Build history of the part. All positions in model axes, mm. A direction names the side the tool comes from. Give positions to 0.01 mm unless a question says otherwise; leave off trailing zeros. Write each loop counter-clockwise with the first axis right and the second up, starting at its lowest first coordinate (ties: lowest second). Pieces come first, ordered by that corner, then holes.
Autodesk Inventor part; units mm, degrees
ref_plane "YZ Plane" through (0, 0, 0) normal (1, 0, 0) x (0, 1, 0)
ref_plane "XZ Plane" through (0, 0, 0) normal (0, 1, 0) x (-1, 0, 0)
ref_plane "XY Plane" through (0, 0, 0) normal (0, 0, 1) x (1, 0, 0)
sketch "Sketch1" plane through (0, 0, 0) normal (0, 1, 0) x (-1, 0, 0)
  line L0 (-24.2, -24.2) -> (24.2, -24.2)
  line L1 (24.2, -24.2) -> (24.2, 24.2)
  line L2 (24.2, 24.2) -> (-24.2, 24.2)
  line L3 (-24.2, 24.2) -> (-24.2, -24.2)
  point P0 (0, 0)
  point P1 (0, 24.2)
  point P2 (-24.2, 0)
  dimension "d0" = 48.4
  dimension "d2" = 48.4
extrude "Extrusion1" add sketch "Sketch1" along normal blind 45
sketch "Sketch2" plane through (0, 45, 0) normal (0, 1, 0) x (1, 0, 0)
  circle A0 centre (0, 0) radius 21
  dimension "d5" = 42
extrude "Extrusion2" add sketch "Sketch2" along normal blind 12.5
sketch "Sketch3" plane through (0, 57.5, 0) normal (0, 1, 0) x (1, 0, 0)
  circle A0 centre (0, 0) radius 21
  circle A1 centre (0, 0) radius 20.1325
extrude "Extrusion3" add sketch "Sketch3" along normal blind 9 contours A1
chamfer "Chamfer1" distance 2 distance2 9 1 edges at (-20.1325, 66.5, 0) measured on face at (-5.7471, 66.5, 1.5127)
sketch "Sketch4" plane through (0, 66.5, 0) normal (0, 1, 0) x (1, 0, 0)
  circle A0 centre (0, 0) radius 18.1325
extrude "Extrusion4" add sketch "Sketch4" along normal blind 9
sketch "Sketch5" plane through (0, 45, 0) normal (0, 1, 0) x (1, 0, 0)
  circle A0 centre (0, 0) radius 21
  line L0 (24.2, 24.2) -> (-24.2, 24.2)
  line L1 (-4.5, 24.2) -> (4.5, 24.2)
  line L2 (4.5, 24.2) -> (4.5, 14)
  line L3 (4.5, 14) -> (-4.5, 14)
  line L4 (-4.5, 14) -> (-4.5, 24.2)
  dimension "d16" = 9
  dimension "d18" = 4.5
extrude "Extrusion5" add sketch "Sketch5" along normal blind 20 contours L2 L3 L4 A0 | A0 L4 L0 L2 picked at (0.5035, 16.3152)
sketch "Sketch6" plane through (0, 0, 0) normal (0, -1, 0) x (1, 0, 0)
  line L0 (24.2, -24.2) -> (-24.2, -24.2)
  line L1 (24.2, 24.2) -> (24.2, -24.2)
  line L2 (-24.2, 24.2) -> (24.2, 24.2)
  line L3 (-24.2, -24.2) -> (-24.2, 24.2)
  point P0 (0, 0)
  point P1 (19.2, 19.2)
  point P2 (-19.2, -19.2)
  dimension "d21" = 5
  dimension "d22" = 5
  dimension "d23" = 5
  dimension "d24" = 5
hole "Hole1" at (19.2, 0, 19.2) at (-19.2, 0, -19.2) direction (0, 1, 0) diameter 2.5 depth 8 tip angle 118
sketch "Sketch7" plane through (-24.2, 0, -24.2) normal (-1, 0, 0) x (0, 0, 1)
  line L0 (38, 6) -> (44, 6)
  line L1 (44, 6) -> (44, 3)
  line L2 (44, 3) -> (38, 3)
  line L3 (38, 3) -> (38, 6)
  point P0 (24.2, 0)
extrude "Extrusion6" cut sketch "Sketch7" against normal blind 5
fillet "Fillet1" radius 2 2 edges at (-21.7, 6, 13.8) (-21.7, 6, 19.8)
properties part number "Lidar"
1. Drop flat-ended pins along their axis: pin 1 (4 mm diameter, centred on y = 51.5, z = -5, fed in from -X); pin 2 (4 mm diameter, centred on x = 13, y = 50, fed in from -Z); pin 3 (1.5 mm diameter, centred on y = 4.5, z = 16, fed in from -X); pin 4 (2 mm diameter, centred on x = -21, z = 17.5, fed in from -Y). Give the stop position or say it passes through.
2. 3-axis set-ups, long thin cutter, end or side, ignore diameter. For faces 1 (the face through (-20.254, 4.056, -19.872)), 2 (the face through (-4.5, 57, -22)), 3 (the face through (-19.2, 5, 17)), 4 (the face through (-18.115, 70.937, 0.797)): which of +Z, -Z, +X, -X, +Y, -Y reach the whole face in a straight line?
3. Mould opens along Z. For faces 5 (the face through (-21.66, 5.43, 19.2)), 6 (the face through (19.35, 8.62, 19.36)), 7 (the face through (0, 22, 24.2)), 8 (the face through (0, 0, 0)) say: pulls with the +Z half, pulls with the -Z half, needs draft (parallel to the pull), parting line crosses it, or undercut.
4. Saw through at B-B on y = 56.5. Give the cut face in (x, z), plus the area to 3 significant figures.
5. Drill centre lines: line 1 along Z through (x, y) = (19, 5); line 2 along X through (y, z) = (4, -19). Where is each one in solid material? Low to high.
Outcome:
1. pin 1: stops at x = -20.78
1. pin 2: stops at z = -17.89
1. pin 3: stops at x = -19.2
1. pin 4: stops at y = 0
2. face 1: -Y
2. face 2: -Z, -X, +Y
2. face 3: -X
2. face 4: +Y
3. face 5: undercut
3. face 6: undercut
3. face 7: pulls with the +Z half
3. face 8: needs draft
4. outline: (-4.5, -24.2) - (4.5, -24.2) - (4.5, -20.51) arc R21 ccw (long way) to (-4.5, -20.51) - close
4. area: 1,420 mm2
5. line 1: z = -24.2 to 17.97, 20.43 to 24.2
5. line 2: x = -24.2 to -20.43, -17.97 to 24.2
